Geometry: final body of the model. Coordinates: model frame, mm. A direction names the side the tool comes from. Give positions to 0.01 mm unless a question says otherwise; leave off trailing zeros. Write each loop counter-clockwise with the first axis right and the second up, starting at its lowest first coordinate (ties: lowest second). Pieces come first, ordered by that corner, then holes. Notation, with made-up numbers: M 51,49 L 75,49 A12 ccw 75,63 Z; hole C 2.25,26 d3. An arc over 180 degrees is marked long. Use a Markdown table: item, result. Add a question column.
1) Section D-D on z = -24. Return the cut outline in (x, y).
2) Section B-B on y = -1. Return the cut outline in (x, z).
3) Section A-A on z = 0. Return the cut outline in (x, y).
4) Pin query (flat end, axial travel): pin 1 (2.5 mm diameter, centred on y = -7, z = -25, fed in from +X); pin 2 (1.5 mm diameter, centred on x = -24.5, y = -3.5, fed in from +Z); pin 3 (3 mm diameter, centred on x = -8, y = -1, fed in from +Z); pin 4 (1.5 mm diameter, centred on y = -1.5, z = -30.5, fed in from -X). Return the tip coordinate at first contact, or that it passes through.
5) Line query: line 1 (X direction, y = 0.9, z = 0); line 2 (Z direction, x = 26, y = -1.75). Output: solid intervals per line, ascending.
6) Section C-C on x = 19.5. Return the cut outline in (y, z).
7) Draft query along X for faces 5 (the flat face through (22.5, -5, 25)), 6 (the flat face through (-27.5, -5, 25)), 7 (the cylindrical face through (8.431, 0.986, 37.966)), 8 (the flat face through (25, -5, -27.5)). Return one class per face: +X half, -X half, draft (parallel to the pull), parting line (faces both ways), or undercut.
8) Set-up query: faces 1 (the flat face through (22.5, -5, -25)), 2 (the flat face through (-25, -5, 27.5)), 3 (the flat face through (-25, -5, 22.5)), 4 (the flat face through (-27.5, -5, -25)). Return all of +Z, -Z, +X, -X, +Y, -Y with unobstructed straight access to the full face (end or side cutting, diameter ignored); none if empty.
Autodesk Inventor part; units mm, degrees
ref_plane "YZ Plane" through (0, 0, 0) normal (1, 0, 0) x (0, 1, 0)
ref_plane "XZ Plane" through (0, 0, 0) normal (0, 1, 0) x (-1, 0, 0)
ref_plane "XY Plane" through (0, 0, 0) normal (0, 0, 1) x (1, 0, 0)
sketch "Szkic1" plane through (0, 0, 0) normal (0, 1, 0) x (-1, 0, 0)
  line L0 (-25, -25) -> (25, -25)
  line L1 (25, -25) -> (25, 25)
  line L2 (25, 25) -> (-25, 25)
  line L3 (-25, 25) -> (-25, -25)
  line L4 (-25, -25) -> (25, 25) construction
  line L5 (25, -25) -> (-25, 25) construction
  line L6 (22.5, 22.5) -> (27.5, 22.5)
  line L7 (27.5, 22.5) -> (27.5, 27.5)
  line L8 (27.5, 27.5) -> (22.5, 27.5)
  line L9 (22.5, 27.5) -> (22.5, 22.5)
  line L10 (22.5, 22.5) -> (27.5, 27.5) construction
  line L11 (27.5, 22.5) -> (22.5, 27.5) construction
  line L12 (27.5, -27.5) -> (22.5, -27.5)
  line L13 (22.5, -27.5) -> (22.5, -22.5)
  line L14 (22.5, -22.5) -> (27.5, -22.5)
  line L15 (27.5, -22.5) -> (27.5, -27.5)
  line L16 (27.5, -27.5) -> (22.5, -22.5) construction
  line L17 (22.5, -27.5) -> (27.5, -22.5) construction
  line L18 (-27.5, -22.5) -> (-22.5, -22.5)
  line L19 (-22.5, -22.5) -> (-22.5, -27.5)
  line L20 (-22.5, -27.5) -> (-27.5, -27.5)
  line L21 (-27.5, -27.5) -> (-27.5, -22.5)
  line L22 (-27.5, -22.5) -> (-22.5, -27.5) construction
  line L23 (-22.5, -22.5) -> (-27.5, -27.5) construction
  line L24 (-27.5, 27.5) -> (-22.5, 27.5)
  line L25 (-22.5, 27.5) -> (-22.5, 22.5)
  line L26 (-22.5, 22.5) -> (-27.5, 22.5)
  line L27 (-27.5, 22.5) -> (-27.5, 27.5)
  line L28 (-27.5, 27.5) -> (-22.5, 22.5) construction
  line L29 (-22.5, 27.5) -> (-27.5, 22.5) construction
  circle A0 centre (0, 0) radius 35.3553
  circle A1 centre (0, 0) radius 38.8909
  circle A2 centre (0, 0) radius 31.8198
  point P0 (-19.685, 25)
  point P1 (19.685, 25)
  point P2 (25, 19.685)
  point P3 (25, -19.685)
  point P4 (19.685, -25)
  point P5 (-19.685, -25)
  point P6 (-25, -19.685)
  point P7 (-25, 19.685)
  dimension "d14" = 63.6396
  dimension "d0" = 50
  dimension "d1" = 50
  dimension "d2" = 5
  dimension "d3" = 5
  dimension "d4" = 5
  dimension "d5" = 5
  dimension "d6" = 5
  dimension "d7" = 5
  dimension "d8" = 5
  dimension "d9" = 5
extrude "Wyciągnięcie proste1" add sketch "Szkic1" along normal blind 2 contours L3 L18 L19 L0 | A0 L18 L3 | A0 L19 L20 L21 L18 | L0 L19 A0 | L19 A2 L0 | L0 A2 L13 A0 L19 | L18 A0 L26 L3 A2 | L3 A2 L18 | L18 L21 A1 L27 L26 A0 | A0 L13 L12 A1 L20 L19 | A0 L3 L26 | L26 L27 L24 L25 A0 | A0 L14 L15 L12 L13 | L13 L0 A0 | A2 L13 L0 | L3 L26 A2 | L3 L2 L25 L26 | A0 L25 L2 | L13 L14 L1 L0 | L1 L14 A0 | A2 L1 L14 | L25 L2 A2 | A1 L8 L9 A0 L25 L24 | L15 L14 A0 L6 L7 A1 | L25 A0 L9 L2 A2 | L1 A2 L6 A0 L14 | L7 L6 A0 L9 L8 | A0 L2 L9 | A2 L6 L1 | L2 L9 A2 | L2 L1 L6 L9 | A0 L6 L1
extrude "Wyciągnięcie proste2" add sketch "Szkic1" against normal blind 10 contours L3 L18 L19 L0 | A0 L18 L3 | A0 L19 L20 L21 L18 | L0 L19 A0 | A0 L3 L26 | L26 L27 L24 L25 A0 | A0 L14 L15 L12 L13 | L13 L0 A0 | L3 L2 L25 L26 | A0 L25 L2 | L13 L14 L1 L0 | L1 L14 A0 | L7 L6 A0 L9 L8 | A0 L2 L9 | L2 L1 L6 L9 | A0 L6 L1
equation "\"d7\" = d6"
properties part number "Tarcza_Podkładka" material "Polietylen o dużej gęstości"
Found:
| question | item | result |
|---|---|---|
| 1 | outline | M -30.6,0 L -27.5,0 L -27.5,-10 L -22.5,-10 L -22.5,0 L -20.89,0 L -20.89,2 L -30.6,2 Z; M 20.89,0 L 22.5,0 L 22.5,-10 L 27.5,-10 L 27.5,0 L 30.6,0 L 30.6,2 L 20.89,2 Z |
| 2 | outline | M -27.5,-27.5 L -22.5,-27.5 L -22.5,-22.5 L -27.5,-22.5 Z; M -27.5,22.5 L -22.5,22.5 L -22.5,27.5 L -27.5,27.5 Z; M 22.5,-27.5 L 27.5,-27.5 L 27.5,-22.5 L 22.5,-22.5 Z; M 22.5,22.5 L 27.5,22.5 L 27.5,27.5 L 22.5,27.5 Z |
| 3 | outline | M -38.89,0 L -31.82,0 L -31.82,2 L -38.89,2 Z; M 31.82,0 L 38.89,0 L 38.89,2 L 31.82,2 Z |
| 4 | pin 1 | x = 27.5 |
| 4 | pin 2 | z = 27.5 |
| 4 | pin 3 | z = 38.28 |
| 4 | pin 4 | through |
| 5 | line 1 | -38.89 to -31.82, 31.82 to 38.89 |
| 5 | line 2 | -27.5 to -22.5, 22.5 to 27.5 |
| 6 | outline | M 0,-33.65 L 2,-33.65 L 2,-25.14 L 0,-25.14 Z; M 0,25.14 L 2,25.14 L 2,33.65 L 0,33.65 Z |
| 7 | face 5 | undercut |
| 7 | face 6 | -X half |
| 7 | face 7 | parting line |
| 7 | face 8 | draft |
| 8 | face 1 | +Z, -Z, -Y |
| 8 | face 2 | +Z, +X, -X, -Y |
| 8 | face 3 | +X, -X, -Y |
| 8 | face 4 | +Z, -Z, -X, -Y |
